from build123d import *

# Parameters (mm, degrees)
SKETCH1_W           = 158
SKETCH1_H           = 56
BOSS_EXTRUDE1_DEPTH = 17
SKETCH8_W           = 13.6
SKETCH8_H           = 12
BOSS_EXTRUDE2_DEPTH = 6
SKETCH2_W           = 36
SKETCH2_H           = 36
CUT_EXTRUDE1_DEPTH  = 11.5
SKETCH3_W           = 26
SKETCH3_H           = 26
CUT_EXTRUDE2_DEPTH  = 3
CUT_EXTRUDE3_REACH  = 88.286
SKETCH4_R           = 9.5
SKETCH5_R           = 2.6
CUT_EXTRUDE4_DEPTH  = 4.5
CUT_EXTRUDE5_REACH  = 87.522
FILLET1_R           = 3
FILLET2_R           = 1
FILLET3_R           = 1
FILLET4_R           = 1
FILLET5_R           = 0.5


with BuildPart() as part:
    # Sketch1 → Boss-Extrude1 (new body)
    with BuildSketch(Plane(origin=(0, 0, 0), x_dir=(1, 0, 0), z_dir=(0, 1, 0))):
        Rectangle(SKETCH1_W, SKETCH1_H)
    extrude(amount=BOSS_EXTRUDE1_DEPTH)

    # Sketch8 → Boss-Extrude2 (add)
    with BuildSketch(Plane(origin=(0, 17, 0), x_dir=(1, 0, 0), z_dir=(0, 1, 0))):
        with Locations((0, -22)):
            Rectangle(SKETCH8_W, SKETCH8_H)
    extrude(amount=BOSS_EXTRUDE2_DEPTH)

    # Sketch2 → Cut-Extrude1 (cut)
    with BuildSketch(Plane(origin=(0, 17, 0), x_dir=(1, 0, 0), z_dir=(0, 1, 0))):
        with Locations((-51, 0)):
            Rectangle(SKETCH2_W, SKETCH2_H)
        with Locations((51, 0)):
            Rectangle(SKETCH2_W, SKETCH2_H)
    extrude(amount=-CUT_EXTRUDE1_DEPTH, mode=Mode.SUBTRACT)

    # Sketch3 → Cut-Extrude2 (cut)
    with BuildSketch(Plane(origin=(0, 5.5, 0), x_dir=(1, 0, 0), z_dir=(0, 1, 0))):
        with Locations((51, 0)):
            Rectangle(SKETCH3_W, SKETCH3_H)
        with Locations((-51, 0)):
            Rectangle(SKETCH3_W, SKETCH3_H)
    extrude(amount=-CUT_EXTRUDE2_DEPTH, mode=Mode.SUBTRACT)

    # Sketch4 → Cut-Extrude3 (cut, up to next)
    with BuildSketch(Plane(origin=(0, 2.5, 0), x_dir=(1, 0, 0), z_dir=(0, 1, 0)), mode=Mode.PRIVATE) as cut_extrude3_sk1:
        with Locations(Location((-51, 0, 0), (0, 0, 270))):
            Circle(SKETCH4_R)
    cut_extrude3_tool1 = extrude(cut_extrude3_sk1.sketch, amount=-CUT_EXTRUDE3_REACH, mode=Mode.PRIVATE) & part.part
    # Sketch4 → Cut-Extrude3 (cut, up to next)
    with BuildSketch(Plane(origin=(0, 2.5, 0), x_dir=(1, 0, 0), z_dir=(0, 1, 0)), mode=Mode.PRIVATE) as cut_extrude3_sk2:
        with Locations(Location((51, 0, 0), (0, 0, 270))):
            Circle(SKETCH4_R)
    cut_extrude3_tool2 = extrude(cut_extrude3_sk2.sketch, amount=-CUT_EXTRUDE3_REACH, mode=Mode.PRIVATE) & part.part
    add(cut_extrude3_tool1.solids().sort_by_distance((-51, 2.5, 0))[0], mode=Mode.SUBTRACT)
    add(cut_extrude3_tool2.solids().sort_by_distance((51, 2.5, 0))[0], mode=Mode.SUBTRACT)

    # Sketch5 → Cut-Extrude4 (cut)
    with BuildSketch(Plane(origin=(0, 17, 0), x_dir=(1, 0, 0), z_dir=(0, 1, 0))):
        with Locations(Location((-73.5, 22.5, 0), (0, 0, 270))):
            Circle(SKETCH5_R)
        with Locations(Location((73.5, 22.5, 0), (0, 0, 90))):
            Circle(SKETCH5_R)
        with Locations(Location((73.5, -22.5, 0), (0, 0, 270))):
            Circle(SKETCH5_R)
        with Locations(Location((-73.5, -22.5, 0), (0, 0, 90))):
            Circle(SKETCH5_R)
    extrude(amount=-CUT_EXTRUDE4_DEPTH, mode=Mode.SUBTRACT)

    # Sketch6 → Cut-Extrude5 (cut, up to next)
    with BuildSketch(Plane(origin=(0, 17, 0), x_dir=(1, 0, 0), z_dir=(0, 1, 0)), mode=Mode.PRIVATE) as cut_extrude5_sk1:
        with BuildLine():
            Line((-20, 6.4), (20, 6.4))
            ThreePointArc((20, 6.4), (21.6, 4.8), (20, 3.2))
            Line((20, 3.2), (-20, 3.2))
            ThreePointArc((-20, 3.2), (-21.6, 4.8), (-20, 6.4))
        make_face()
    cut_extrude5_tool1 = extrude(cut_extrude5_sk1.sketch, amount=-CUT_EXTRUDE5_REACH, mode=Mode.PRIVATE) & part.part
    # Sketch6 → Cut-Extrude5 (cut, up to next)
    with BuildSketch(Plane(origin=(0, 17, 0), x_dir=(1, 0, 0), z_dir=(0, 1, 0)), mode=Mode.PRIVATE) as cut_extrude5_sk2:
        with BuildLine():
            Line((-20, 16), (20, 16))
            ThreePointArc((20, 16), (21.6, 14.4), (20, 12.8))
            Line((20, 12.8), (-20, 12.8))
            ThreePointArc((-20, 12.8), (-21.6, 14.4), (-20, 16))
        make_face()
    cut_extrude5_tool2 = extrude(cut_extrude5_sk2.sketch, amount=-CUT_EXTRUDE5_REACH, mode=Mode.PRIVATE) & part.part
    # Sketch6 → Cut-Extrude5 (cut, up to next)
    with BuildSketch(Plane(origin=(0, 17, 0), x_dir=(1, 0, 0), z_dir=(0, 1, 0)), mode=Mode.PRIVATE) as cut_extrude5_sk3:
        with BuildLine():
            Line((-20, -6.4), (20, -6.4))
            ThreePointArc((20, -6.4), (21.6, -4.8), (20, -3.2))
            Line((20, -3.2), (-20, -3.2))
            ThreePointArc((-20, -3.2), (-21.6, -4.8), (-20, -6.4))
        make_face()
    cut_extrude5_tool3 = extrude(cut_extrude5_sk3.sketch, amount=-CUT_EXTRUDE5_REACH, mode=Mode.PRIVATE) & part.part
    # Sketch6 → Cut-Extrude5 (cut, up to next)
    with BuildSketch(Plane(origin=(0, 17, 0), x_dir=(1, 0, 0), z_dir=(0, 1, 0)), mode=Mode.PRIVATE) as cut_extrude5_sk4:
        with BuildLine():
            Line((-20, -16), (20, -16))
            ThreePointArc((20, -16), (21.6, -14.4), (20, -12.8))
            Line((20, -12.8), (-20, -12.8))
            ThreePointArc((-20, -12.8), (-21.6, -14.4), (-20, -16))
        make_face()
    cut_extrude5_tool4 = extrude(cut_extrude5_sk4.sketch, amount=-CUT_EXTRUDE5_REACH, mode=Mode.PRIVATE) & part.part
    add(cut_extrude5_tool1.solids().sort_by_distance((0, 17, -4.8))[0], mode=Mode.SUBTRACT)
    add(cut_extrude5_tool2.solids().sort_by_distance((0, 17, -14.4))[0], mode=Mode.SUBTRACT)
    add(cut_extrude5_tool3.solids().sort_by_distance((0, 17, 4.8))[0], mode=Mode.SUBTRACT)
    add(cut_extrude5_tool4.solids().sort_by_distance((0, 17, 14.4))[0], mode=Mode.SUBTRACT)

    # Fillet1
    fillet1_edges = [part.edges().sort_by_distance(p)[0] for p in [
        (79, 8.5, 28),
        (-79, 8.5, 28),
        (-79, 8.5, -28),
        (79, 8.5, -28),
    ]]
    fillet(fillet1_edges, radius=FILLET1_R)

    # Fillet2
    fillet2_edges = [part.edges().sort_by_distance(p)[0] for p in [
        (-51, 2.5, -9.5),
        (51, 2.5, -9.5),
    ]]
    fillet(fillet2_edges, radius=FILLET2_R)

    # Fillet3
    fillet3_edges = [part.edges().sort_by_distance(p)[0] for p in [
        (38, 5.5, 0),
        (51, 5.5, 13),
        (64, 5.5, 0),
        (51, 5.5, -13),
        (-51, 5.5, -13),
        (-64, 5.5, 0),
        (-51, 5.5, 13),
        (-38, 5.5, 0),
    ]]
    fillet(fillet3_edges, radius=FILLET3_R)

    # Fillet4
    fillet4_edges = [part.edges().sort_by_distance(p)[0] for p in [
        (-33, 17, 0),
        (-51, 17, -18),
        (-69, 17, 0),
        (-51, 17, 18),
        (69, 17, 0),
        (51, 17, -18),
        (33, 17, 0),
        (51, 17, 18),
    ]]
    fillet(fillet4_edges, radius=FILLET4_R)

    # Fillet5
    fillet5_edges = [part.edges().sort_by_distance(p)[0] for p in [
        (0, 23, 28),
        (0, 23, 16),
    ]]
    fillet(fillet5_edges, radius=FILLET5_R)


solid = part.part
Input: part model. Units: mm. Frame: model coordinates. A direction names the side the tool comes from. Round coordinates to 2 decimals unless told otherwise and drop trailing zeros. Order: outer loops, then holes, each group sorted by start corner. A loop starts at its lowest first (then second) coordinate and runs counter-clockwise, first axis right, second up. Notation, with made-up numbers: (14, -29) - (25, -29) arc R20 cw to (25, 5) - close; hole circle Ø7 at (-34.75, 74). An arc over 180 degrees is marked (long way). Answer as a JSON object with one key per item and string values. Group by question number.
(1) Draft query along X for faces 1 (the face through (-79, 8, 0)), 2 (the face through (-76.078, 14.782, 22.838)), 3 (the face through (-1, 0, 0)). Return one class per face: released by +X, released by -X, zero draft, split by the parting line, or undercut.
(2) Cut plane B-B (y = 7.5). Count the separate pieces of the cut face and the enclosed holes in it, then the cut area to 3 significant figures.
(3) Material intervals for probe 1 along X at (y, z) = (10, 2); probe 2 along X at (y, z) = (13.95, -22.5); probe 3 along X at (y, z) = (8, 4.5), sorted ascending. Write a range as from..to.
(4) Pin query (flat end, axial travel): P1, Ø2.5, axis at x = -73.5, z = 23.5, coming from the +Y side; P2, Ø11, axis at x = -51, z = 0, coming from the +Y side; P3, Ø3, axis at x = 5.5, z = 9, coming from the +Y side; P4, Ø21, axis at x = -49.5, z = -2, coming from the +Y side. Return the tip coordinate at first contact, or that it passes through.
(5) Reachability of faces 4 (the face through (-78.14, 8.62, 27.1)), 5 (the face through (-51, 11, 18)), 6 (the face through (21.6, 8.6, 14.4)), 7 (the face through (-6.8, 20, 22)) from +Z, -Z, +X, -X, +Y, -Y: full face, straight path, thin tool, end or side. Return the list, or none.
(6) Cut plane A-A (x = 51). Return loops of the section in (y, z), then the cut area to 3 significant figures.
(7) Cut plane C-C (x = 12.5). Return loops of the section in (y, z).
Here are the results:
{
 "1": {"face 1": "released by -X", "face 2": "undercut", "face 3": "zero draft"},
 "2": {"separate pieces": "1", "enclosed holes": "6", "area": "5,700 mm^2"},
 "3": {"probe 1": "x = -79..-69, -33..33, 69..79", "probe 2": "x = -79..-76.1, -70.9..70.9, 76.1..79", "probe 3": "x = -79..-69, -33..-21.57, 21.57..33, 69..79"},
 "4": {"P1": "stops at y = 12.5", "P2": "passes through", "P3": "stops at y = 17", "P4": "stops at y = 2.5"},
 "5": {"face 4": "+Z, -X, +Y, -Y", "face 5": "+Y", "face 6": "+Y, -Y", "face 7": "+Z, -Z, -X, +Y"},
 "6": {"outline": "(0, -28) - (17, -28) - (17, -19) arc R1 ccw to (16, -18) - (5.5, -18) - (5.5, -14) arc R1 ccw to (4.5, -13) - (2.5, -13) - (2.5, -10.5) arc R1 ccw to (1.5, -9.5) - (0, -9.5) - close; (0, 9.5) - (1.5, 9.5) arc R1 ccw to (2.5, 10.5) - (2.5, 13) - (4.5, 13) arc R1 ccw to (5.5, 14) - (5.5, 18) - (16, 18) arc R1 ccw to (17, 19) - (17, 28) - (0, 28) - close", "area": "411 mm^2"},
 "7": {"outline": "(0, -28) - (17, -28) - (17, -16) - (0, -16) - close; (0, -12.8) - (17, -12.8) - (17, -6.4) - (0, -6.4) - close; (0, -3.2) - (17, -3.2) - (17, 3.2) - (0, 3.2) - close; (0, 6.4) - (17, 6.4) - (17, 12.8) - (0, 12.8) - close; (0, 16) - (17, 16) - (17, 28) - (0, 28) - close"}
}
